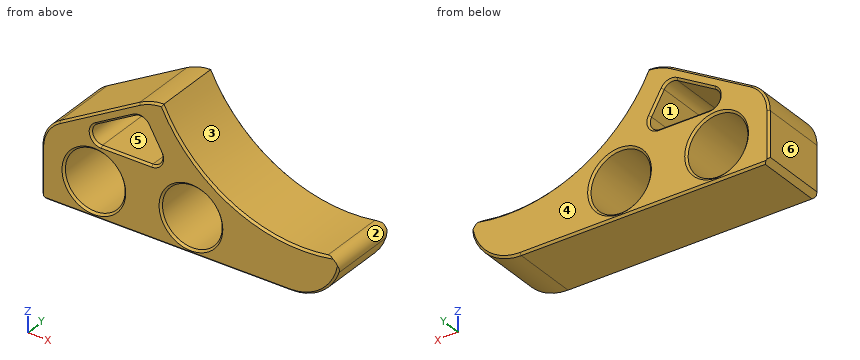
from build123d import *

# Parameters (mm, degrees)
F0_R        = 30
F1_DEPTH    = 35
F2_T1_DEPTH = 320
F3_SIZE     = 2
F4_T1_DEPTH = 91.7168298797
F5_T1_DEPTH = 146.5537481792


# Not quite as in the source:
# - a fillet or chamfer that OpenCascade refuses, or shapes differently, is made with other operations: its cross-section is extruded or revolved along the edge and cut away or added


with BuildPart() as f1:
    # F0 (on Front) → F1 (new body, symmetric)
    with BuildSketch(Plane.XZ):
        with BuildLine():
            Line((-150, -35), (150, -35))
            Line((150, -35), (150, 14.7927405784))
            ThreePointArc((150, 14.7927405784), (45.9749646372, 24.7257009589), (-28.4932742745, 98.0356803447))
            ThreePointArc((-28.4932742745, 98.0356803447), (-40.8686708706, 96.1996481654), (-52.4008673876, 91.3488854864))
            Line((-52.4008673876, 91.3488854864), (-132.5, 45.1036297108))
            ThreePointArc((-132.5, 45.1036297108), (-145.3108891325, 32.2927405784), (-150, 14.7927405784))
            Line((-150, 14.7927405784), (-150, -35))
        make_face()
        with Locations((-97.5, 0)):
            Circle(F0_R, mode=Mode.SUBTRACT)
        Circle(F0_R, mode=Mode.SUBTRACT)
        with BuildLine():
            ThreePointArc((-90.1794919243, 36.443375673), (-99.8387501872, 43.8551852219), (-95.1794919243, 55.1036297108))
            Line((-95.1794919243, 55.1036297108), (-57.1537916494, 77.0577780006))
            ThreePointArc((-57.1537916494, 77.0577780006), (-49.5656011984, 78.0567822257), (-43.4935376116, 73.3975239628))
            Line((-43.4935376116, 73.3975239628), (-30.8183041866, 51.443375673))
            ThreePointArc((-30.8183041866, 51.443375673), (-30.8183041866, 41.443375673), (-39.4785582245, 36.443375673))
            Line((-39.4785582245, 36.443375673), (-90.1794919243, 36.443375673))
        make_face(mode=Mode.SUBTRACT)
    extrude(amount=F1_DEPTH, both=True)

    # F2: fillet of radius 50 on 1 edges, made by hand

    # F2_s2 → F2_t1 (cut)
    with BuildSketch(Plane.XZ.offset(-160)):
        with BuildLine():
            ThreePointArc((150, 15), (135.3553390593, -20.3553390593), (100, -35))
            Line((100, -35), (150, -35))
            Line((150, -35), (150, 15))
        make_face()
    extrude(amount=F2_T1_DEPTH, mode=Mode.SUBTRACT)

    # F3
    f3_edges = [f1.edges().sort_by_distance(p)[0] for p in [
        (135.281947, -35, -20.428579),
        (-25, -35, -35),
        (-150, -35, -10.10363),
        (-145.310889, -35, 32.292741),
        (-92.450434, -35, 68.226258),
        (-40.868671, -35, 96.199648),
        (45.974764, -35, 24.725795),
        (-127.5, -35, 0),
        (-30, -35, 0),
        (-99.83875, -35, 43.855185),
        (-64.829025, -35, 36.443376),
        (-76.166642, -35, 66.080704),
        (-30.818304, -35, 41.443376),
        (-49.565601, -35, 78.056782),
        (-37.155921, -35, 62.42045),
        (135.281947, 35, -20.428579),
        (-25, 35, -35),
        (-150, 35, -10.10363),
        (-145.310889, 35, 32.292741),
        (-92.450434, 35, 68.226258),
        (-40.868671, 35, 96.199648),
        (45.974764, 35, 24.725795),
        (-127.5, 35, 0),
        (-30, 35, 0),
        (-99.83875, 35, 43.855185),
        (-64.829025, 35, 36.443376),
        (-76.166642, 35, 66.080704),
        (-30.818304, 35, 41.443376),
        (-49.565601, 35, 78.056782),
        (-37.155921, 35, 62.42045),
    ]]
    chamfer(f3_edges, length=F3_SIZE)

    # F4: chamfer of 5 on 1 edges, made by hand

    # F4_s2 → F4_t1 (cut)
    with BuildSketch(Plane.XZ.offset(-45.8584149398)):
        Polygon((-145, -35), (-150, -30), (-150, -35), align=None)
    extrude(amount=F4_T1_DEPTH, mode=Mode.SUBTRACT)

    # F5: fillet of radius 10 on 1 edges, made by hand

    # F5_s2 → F5_t1 (cut)
    with BuildSketch(Plane.XZ.offset(-73.2768740896)):
        with BuildLine():
            ThreePointArc((136.3119389308, 12.0003957225), (145.5204541724, 8.5629129702), (147.338085728, -1.0967586678))
            ThreePointArc((147.338085728, -1.0967586678), (149.3130103908, 6.7400359449), (149.9995699858, 14.7926326161))
            ThreePointArc((149.9995699858, 14.7926326161), (143.1869943531, 13.243375245), (136.3119389308, 12.0003957225))
        make_face()
    extrude(amount=F5_T1_DEPTH, mode=Mode.SUBTRACT)


solid = f1.part
The listing builds one solid part. Answer for the finished solid, in the listing's coordinates (mm). Face numbers are marked on the shaded views. A direction names the side the tool comes from. Round coordinates to 2 decimals unless told otherwise and drop trailing zeros. Write each loop counter-clockwise with the first axis right and the second up, starting at its lowest first coordinate (ties: lowest second). Pieces come first, ordered by that corner, then holes. Notation, with made-up numbers: (-13.75, -17.75) - (-6.75, -17.75) arc R28 cw to (-6.75, 0.25) - close; hole circle Ø1 at (-32, -11). An arc over 180 degrees is marked (long way). Use one line per item in the form item = value. Start each with the question number.
Item 1: Flat-ended cylindrical pins translate along their axes: pin 1 Ø8 at (y, z) = (22, 57.5) entering from +X; pin 2 Ø12 at (y, z) = (-18.5, 30.5) entering from -X. Find the tip coordinate at first contact, or state that the pin passes through.
Item 2: Determine the mould class of the marked faces 1, 2, 3 and 4 for opening direction Z: +Z half, -Z half, draft (parallel to the pull), parting line (faces both ways), or undercut.
Item 3: A cutting plane is placed at A-A (y = -22.5). Write down the section's boundary in (x, z), plus the area to 3 significant figures.
Item 4: Find the intervals of material crossed by line 1 (X direction, y = -23, z = -1); line 2 (Z direction, x = -97.5, y = -18.5); line 3 (X direction, y = -16.5, z = -4), in increasing order. Write a range as [from, to].
Item 5: A tool of negligible diameter and unlimited length cuts with its end or side. For the marked faces 5 and 6, from which of +Z, -Z, +X, -X, +Y, -Y can it reach the whole face along a straight path? Write none if from no direction.
The answers:
q1.pin_1 = 3.94
q1.pin_2 = -148.63
q2.face_1 = undercut
q2.face_2 = parting line
q2.face_3 = +Z half
q2.face_4 = draft
q3.outline = (-150, -30) - (-145, -35) - (100, -35) arc R50 ccw to (147.34, -1.1) arc R10 ccw to (136.31, 12) arc R156.15 cw to (-28.49, 98.04) arc R50 ccw to (-52.4, 91.35) - (-132.5, 45.1) arc R35 ccw to (-150, 14.79) - close; hole circle Ø60 at (-97.5, 0); hole (-95.18, 55.1) arc R10 ccw to (-90.18, 36.44) - (-39.48, 36.44) arc R10 ccw to (-30.82, 51.44) - (-43.49, 73.4) arc R10 ccw to (-57.15, 77.06) - close; hole circle Ø60 at (0, 0)
q3.area = 15,900 mm^2
q4.line_1 = [-150, -127.48], [-67.52, -29.98], [29.98, 147.37]
q4.line_2 = [-35, -30], [30, 39.63], [53.26, 65.31]
q4.line_3 = [-150, -127.23], [-67.77, -29.73], [29.73, 146.25]
q5.face_5 = +Y, -Y
q5.face_6 = +Z, -Z, -X, +Y, -Y
